Could you check a few things on this model? Use its own coordinates, in mm. A direction names the side the tool comes from. Round coordinates to 2 decimals unless told otherwise and drop trailing zeros. Order: outer loops, then holes, each group sorted by start corner. A loop starts at its lowest first (then second) coordinate and runs counter-clockwise, first axis right, second up. Notation, with made-up numbers: (-1.5, 71.25) - (7.5, 71.25) arc R24 cw to (7.5, 104.25) - close; hole circle Ø11 at (-14, 18). An arc over 180 degrees is marked (long way). Use one line per item in the form item = value.
from build123d import *

# Parameters (mm, degrees)
SALIENTE_EXTRUIR1_DEPTH  = 40
SALIENTE_EXTRUIR2_DEPTH  = 4
CROQUIS3_W               = 70
CROQUIS3_H               = 40
SALIENTE_EXTRUIR3_DEPTH  = 20
SALIENTE_EXTRUIR4_START  = 140
CROQUIS5_W               = 164
CROQUIS5_H               = 70
SALIENTE_EXTRUIR4_DEPTH  = 4
SALIENTE_EXTRUIR5_START  = 164
CROQUIS7_W               = 70
CROQUIS7_H               = 160
SALIENTE_EXTRUIR5_DEPTH  = 4
CROQUIS8_W               = 70
CROQUIS8_H               = 40
SALIENTE_EXTRUIR6_DEPTH  = 20
SALIENTE_EXTRUIR12_DEPTH = 4
CROQUIS11_W              = 24
CROQUIS11_H              = 70
SALIENTE_EXTRUIR13_DEPTH = 4
SALIENTE_EXTRUIR14_START = 40
SALIENTE_EXTRUIR14_DEPTH = 40
SALIENTE_EXTRUIR15_START = 25
SALIENTE_EXTRUIR15_DEPTH = 10
SALIENTE_EXTRUIR16_START = -25
SALIENTE_EXTRUIR16_DEPTH = 10


with BuildPart() as part:
    # Croquis1 → Saliente-Extruir1 (new body)
    with BuildSketch(Plane(origin=(0, 0, 0), x_dir=(0, 0, -1), z_dir=(1, 0, 0))):
        with BuildLine():
            Line((-3, 11.618950039), (-3, 8.485281374))
            ThreePointArc((-3, 8.485281374), (0, -9), (3, 8.485281374))
            Line((3, 8.485281374), (3, 11.618950039))
            ThreePointArc((3, 11.618950039), (0, -12), (-3, 11.618950039))
        make_face()
    extrude(amount=SALIENTE_EXTRUIR1_DEPTH)

    # Croquis2 → Saliente-Extruir2 (add)
    with BuildSketch(Plane.ZY):
        Polygon((-35, 0), (-35, -20), (35, -20), (35, 0), (35, 140), (-35, 140), align=None)
    extrude(amount=SALIENTE_EXTRUIR2_DEPTH)

    # Croquis3 → Saliente-Extruir3 (add)
    with BuildSketch(Plane.ZY.offset(4)):
        with Locations((0, 120)):
            Rectangle(CROQUIS3_W, CROQUIS3_H)
    extrude(amount=SALIENTE_EXTRUIR3_DEPTH)



with BuildPart() as body_2:
    # Croquis5 → Saliente-Extruir4 (new body)
    with BuildSketch(Plane(origin=(0, 0, 0), x_dir=(1, 0, 0), z_dir=(0, 1, 0)).offset(SALIENTE_EXTRUIR4_START)):
        with Locations((82, 0)):
            Rectangle(CROQUIS5_W, CROQUIS5_H)
    extrude(amount=SALIENTE_EXTRUIR4_DEPTH)



with BuildPart() as body_3:
    # Croquis7 → Saliente-Extruir5 (new body)
    with BuildSketch(Plane(origin=(0, 0, 0), x_dir=(0, 0, -1), z_dir=(1, 0, 0)).offset(SALIENTE_EXTRUIR5_START)):
        with Locations((0, 60)):
            Rectangle(CROQUIS7_W, CROQUIS7_H)
    extrude(amount=SALIENTE_EXTRUIR5_DEPTH)

    # Croquis8 → Saliente-Extruir6 (add)
    with BuildSketch(Plane(origin=(168, 0, 0), x_dir=(0, 0, -1), z_dir=(1, 0, 0))):
        with Locations((0, 120)):
            Rectangle(CROQUIS8_W, CROQUIS8_H)
    extrude(amount=SALIENTE_EXTRUIR6_DEPTH)


with BuildPart() as body_2_1:
    add(body_2.part)

    add(body_3.part)  # Saliente-Extruir12 merges body 3
    # Croquis10 → Saliente-Extruir12 (add)
    with BuildSketch(Plane(origin=(0, 140, 0), x_dir=(1, 0, 0), z_dir=(0, 1, 0))):
        Polygon((188, 25), (188, -25), (188, -35), (164, -35), (164, -25), (164, 25), (164, 35), (188, 35), align=None)
    extrude(amount=SALIENTE_EXTRUIR12_DEPTH)


with BuildPart() as part_1:
    add(part.part)

    add(body_2_1.part)  # Saliente-Extruir13 merges body 2
    # Croquis11 → Saliente-Extruir13 (add)
    with BuildSketch(Plane(origin=(0, 140, 0), x_dir=(1, 0, 0), z_dir=(0, 1, 0))):
        with Locations((-12, 0)):
            Rectangle(CROQUIS11_W, CROQUIS11_H)
    extrude(amount=SALIENTE_EXTRUIR13_DEPTH)

    # Croquis12 → Saliente-Extruir14 (add)
    with BuildSketch(Plane.ZY.offset(-164).offset(SALIENTE_EXTRUIR14_START)):
        with BuildLine():
            Line((0, -9), (0, -12))
            ThreePointArc((0, -12), (11.904356355, -1.51205151), (3, 11.618950039))
            Line((3, 11.618950039), (3, 8.485281374))
            ThreePointArc((3, 8.485281374), (8.870387037, -1.521917809), (0, -9))
        make_face()
        with BuildLine():
            ThreePointArc((-3, 11.618950039), (-11.904356355, -1.51205151), (0, -12))
            Line((0, -12), (0, -9))
            ThreePointArc((0, -9), (-8.870387037, -1.521917809), (-3, 8.485281374))
            Line((-3, 8.485281374), (-3, 11.618950039))
        make_face()
    extrude(amount=-SALIENTE_EXTRUIR14_DEPTH)

    # Croquis13 → Saliente-Extruir15 (add)
    with BuildSketch(Plane.XY.offset(SALIENTE_EXTRUIR15_START)):
        Polygon((164, 140), (134, 140), (164, 125), align=None)
        Polygon((0, 140), (30, 140), (0, 125), align=None)
    extrude(amount=SALIENTE_EXTRUIR15_DEPTH)

    # Croquis14 → Saliente-Extruir16 (add)
    with BuildSketch(Plane.XY.offset(SALIENTE_EXTRUIR16_START)):
        Polygon((164, 140), (134, 140), (164, 125), align=None)
        Polygon((0, 140), (30, 140), (0, 125), align=None)
    extrude(amount=-SALIENTE_EXTRUIR16_DEPTH)


solid = part_1.part
Item 1: Imagine slicing it at B-B on x = 149.5. Please give me the cut outline in (y, z), plus the area to 3 significant figures.
Found:
outline = (8.49, -3) arc R9 cw (long way) to (8.49, 3) - (11.62, 3) arc R12 ccw (long way) to (11.62, -3) - close; (132.25, -35) - (144, -35) - (144, 35) - (132.25, 35) - (132.25, 25) - (140, 25) - (140, -25) - (132.25, -25) - close
area = 615 mm2
Item 2: I need wall thicknesses on L1, parallel to Z at x = 23, y = 0; L2, parallel to Y at x = 13, z = 0; L3, parallel to X at y = 103, z = 2.5. Which ranges of each line are inside material? Lowest first, please.
Found:
L1 = -12 to -9, 9 to 12
L2 = -12 to -9, 140 to 144
L3 = -24 to 0, 164 to 188
Item 3: Will these pins go through, and if not, where does the flat tip stop? P1, Ø4.5, axis at x = 143, y = 132, coming from the +Z side; P2, Ø12, axis at y = 1, z = -2.5, coming from the +X side; P3, Ø8, axis at y = 10.5, z = -16.5, coming from the -X side; P4, Ø1.6, axis at x = 143.5, y = 10, coming from the +Z side.
Found:
P1 = through
P2 = 168
P3 = -4
P4 = 7.7
Item 4: If we mould it in two halves opening along Y, with no side actions, what happens to faces 1 (the face through (20, -9, 0)), 2 (the face through (148.8, 132.6, -29.9)), 3 (the face through (9, 136, 25))? For each: released by +Y, released by -Y, zero draft, split by the parting line, or undercut.
Found:
face_1 = undercut
face_2 = released by -Y
face_3 = zero draft
Item 5: Imagine slicing it at A-A on y = 23. Please give me the cut outline in (x, z), plus the area to 3 significant figures.
Found:
outline = (-4, -35) - (0, -35) - (0, 35) - (-4, 35) - close; (164, -35) - (168, -35) - (168, 35) - (164, 35) - close
area = 560 mm2
Item 6: Imagine slicing it at C-C on z = 21. Please give me the cut outline in (x, y), plus the area to 3 significant figures.
Found:
outline = (-24, 100) - (-4, 100) - (-4, -20) - (0, -20) - (0, 140) - (164, 140) - (164, -20) - (168, -20) - (168, 100) - (188, 100) - (188, 144) - (-24, 144) - close
area = 3,730 mm2
Item 7: For faces 4 (the face through (15.2, 132.6, 29.9)), 5 (the face through (9, 136, -25)), 6 (the face through (168, 41, 0)), which set-ups out of +Z, -Z, +X, -X, +Y, -Y let a thin tool reach every point of the face, with its end or its side?
Found:
face_4 = +Z, -Z, -Y
face_5 = -Y
face_6 = +Z, -Z, +X, -Y
Item 8: Imagine slicing it at D-D on y = 0. Please give me the cut outline in (x, z).
Found:
outline = (-4, -35) - (0, -35) - (0, -12) - (40, -12) - (40, -9) - (0, -9) - (0, 9) - (40, 9) - (40, 12) - (0, 12) - (0, 35) - (-4, 35) - close; (124, -12) - (164, -12) - (164, -35) - (168, -35) - (168, 35) - (164, 35) - (164, 12) - (124, 12) - (124, 9) - (164, 9) - (164, -9) - (124, -9) - close
